Check sheet for the drawn part. Datum: minimum x, y, z corner. Units: mm. A direction names the side the tool comes from. Round coordinates to 2 decimals unless told otherwise and drop trailing zeros. Order: outer loops, then holes, each group sorted by start corner. A loop starts at its lowest first (then second) coordinate and runs counter-clockwise, first axis right, second up. Notation, with made-up numbers: (28, 32) -> (81, 32) arc R8 ccw to (81, 37) -> close; hole circle Ø10 at (48, 88). An arc over 180 degrees is marked (long way). Answer as CSV lines item,"result". Start each with the question number.
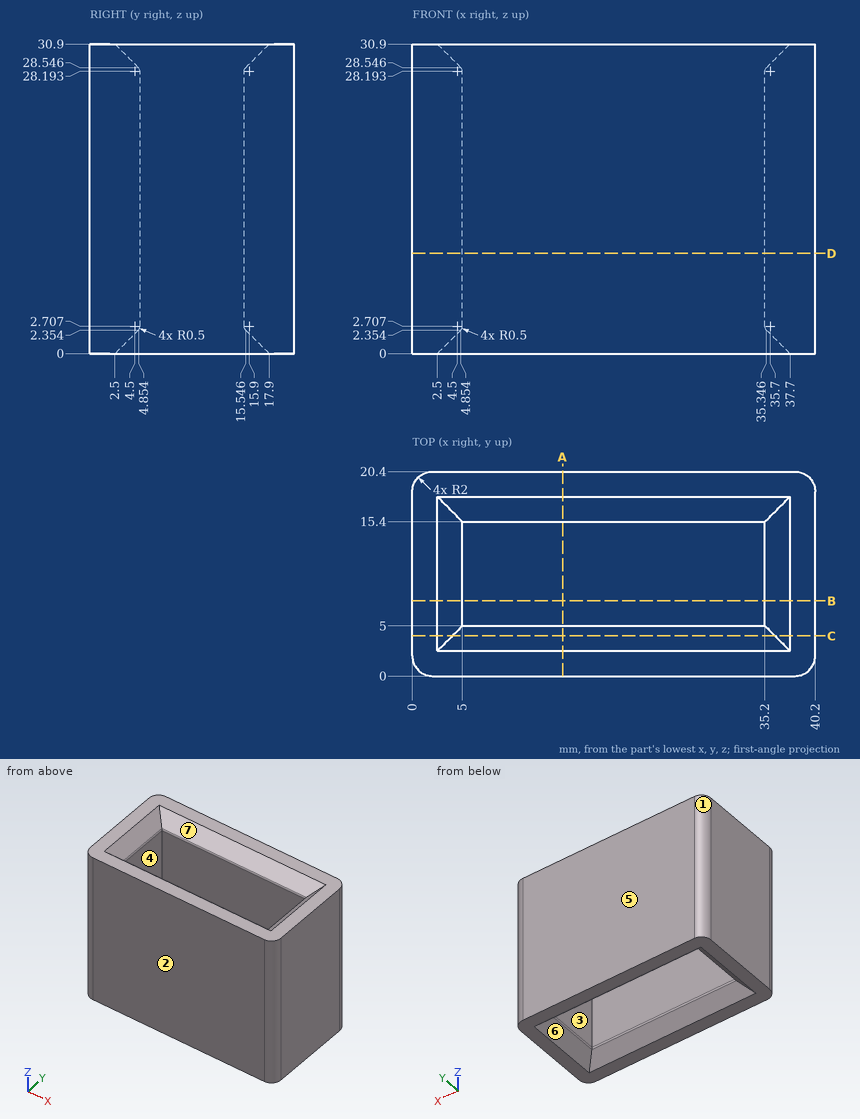
1) Section check A-A on x = 15. Record the cut outline in (y, z).
2) Section check D-D on z = 10. Record the cut outline in (x, y).
3) Section check C-C on y = 4. Record the cut outline in (x, z), then the cut area to 3 significant figures.
4) Mould release check, pull along Y, two halves, no side actions. Record for the marked faces 1, 2 and 3: released by +Y, released by -Y, zero draft, split by the parting line, or undercut.
5) Depth check by flat-ended pin: pin 1 Ø3 at (x, y) = (33, 5) entering from +Z. Enter the tip coordinate at first touch or a pass-through.
6) Section check B-B on y = 7.5. Record the cut outline in (x, z).
7) Access from +Z, -Z, +X, -X, +Y, -Y to the whole of each face (thin tool, end or side, straight path). Record for the marked faces 4, 5, 6 and 7.
8) Material ranges on line 1 along X through (y, z) = (5.5, 21.5); line 2 along Y through (x, z) = (12.5, 9); line 3 along Y through (x, z) = (26.5, 28.5) (1 decimal), recorded low to high.
Solutions:
1,outline,"(0, 0) -> (2.5, 0) -> (4.85, 2.35) arc R0.5 ccw to (5, 2.71) -> (5, 28.19) arc R0.5 ccw to (4.85, 28.55) -> (2.5, 30.9) -> (0, 30.9) -> close; (15.4, 2.71) arc R0.5 ccw to (15.55, 2.35) -> (17.9, 0) -> (20.4, 0) -> (20.4, 30.9) -> (17.9, 30.9) -> (15.55, 28.55) arc R0.5 ccw to (15.4, 28.19) -> close"
2,outline,"(0, 2) arc R2 ccw to (2, 0) -> (38.2, 0) arc R2 ccw to (40.2, 2) -> (40.2, 18.4) arc R2 ccw to (38.2, 20.4) -> (2, 20.4) arc R2 ccw to (0, 18.4) -> close; hole (5, 5) -> (35.2, 5) -> (35.2, 15.4) -> (5, 15.4) -> close"
3,outline,"(0, 0) -> (2.5, 0) -> (4, 1.5) -> (36.2, 1.5) -> (37.7, 0) -> (40.2, 0) -> (40.2, 30.9) -> (37.7, 30.9) -> (36.2, 29.4) -> (4, 29.4) -> (2.5, 30.9) -> (0, 30.9) -> close"
3,area,"1,140 mm^2"
4,face 1,"released by +Y"
4,face 2,"released by -Y"
4,face 3,"undercut"
5,pin 1,"stops at z = 29.9"
6,outline,"(0, 0) -> (2.5, 0) -> (4.85, 2.35) arc R0.5 ccw to (5, 2.71) -> (5, 28.19) arc R0.5 ccw to (4.85, 28.55) -> (2.5, 30.9) -> (0, 30.9) -> close; (35.2, 2.71) arc R0.5 ccw to (35.35, 2.35) -> (37.7, 0) -> (40.2, 0) -> (40.2, 30.9) -> (37.7, 30.9) -> (35.35, 28.55) arc R0.5 ccw to (35.2, 28.19) -> close"
7,face 4,"+Z, -Z"
7,face 5,"+Z, -Z, +X, -X, +Y"
7,face 6,"-Z"
7,face 7,"+Z"
8,line 1,"x = 0 to 5, 35.2 to 40.2"
8,line 2,"y = 0 to 5, 15.4 to 20.4"
8,line 3,"y = 0 to 4.9, 15.5 to 20.4"
